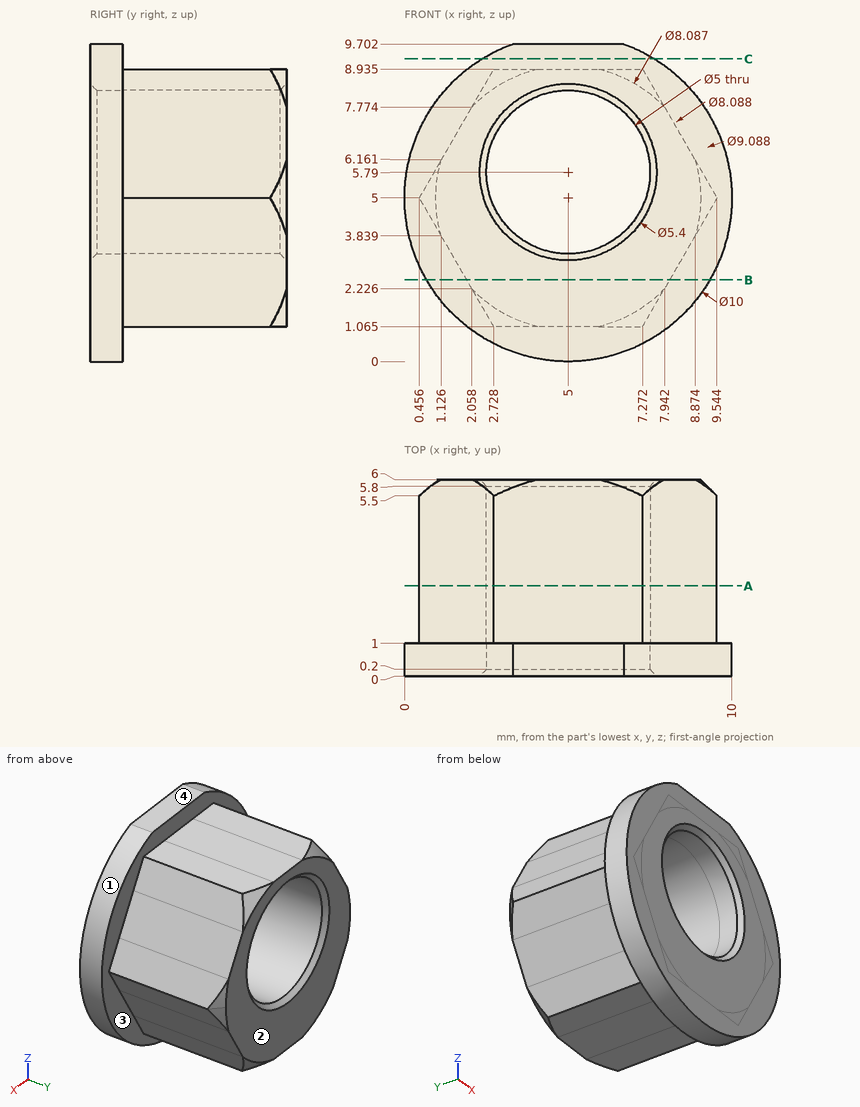
Can you work these out from the drawing? Everything is in mm from the part's minimum corner. A direction names the side the tool comes from. Coordinates: 2 decimals unless noted, no trailing zeros. Loops run counter-clockwise (first coordinate to the right, second up) from the corner with the lowest first, then second, coordinate; pieces in that order, holes last. Notation, with made-up numbers: (7.25, 88) -> (36.25, 88) arc R15 cw to (36.25, 111) -> close; hole circle Ø6 at (4.5, -8). An arc over 180 degrees is marked (long way). Return JSON: item names as keys, results as strings.
1) If we section it at A-A, the plane y = 2.75: Write out the boundary of the cut face in (x, z) (1 decimal).
Results below:
{"outline": "(0.5, 5) -> (1.1, 3.8) -> (2.1, 2.2) -> (2.7, 1.1) -> (7.3, 1.1) -> (7.9, 2.2) -> (8.9, 3.8) -> (9.5, 5) -> (8.9, 6.2) -> (7.9, 7.8) -> (7.3, 8.9) -> (2.7, 8.9) -> (2.1, 7.8) -> (1.1, 6.2) -> close; hole circle Ø5 at (5, 5.8)"}
2) For the marked faces 3 and 4, which set-ups out of +Z, -Z, +X, -X, +Y, -Y let a thin tool reach every point of the face, with its end or its side?
Results below:
{"face 3": "+Y", "face 4": "+Z, +X, -X, +Y, -Y"}
3) Thinking about a two-plate mould opening in Y: for the marked faces 1 and 2, which applies, +Y half, -Y half, draft (parallel to the pull), parting line (faces both ways), or undercut?
Results below:
{"face 1": "draft", "face 2": "+Y half"}
4) If we section it at B-B, the plane z = 2.5: Write out the boundary of the cut face in (x, y).
Results below:
{"outline": "(0.67, 0) -> (9.33, 0) -> (9.33, 1) -> (8.1, 1) -> (8.1, 6) -> (1.9, 6) -> (1.9, 1) -> (0.67, 1) -> close"}
5) I need wall thicknesses on line 1 (X direction, y = 0.5, z = 5.75); line 2 (Z direction, x = 6, y = 1.5) (1 decimal); line 3 (X direction, y = 4.25, z = 4.5) (1 decimal). Which ranges of each line are inside material? Lowest first, please. Write a range as from..to.
Results below:
{"line 1": "0.06..2.5, 7.5..9.94", "line 2": "1.1..3.5, 8.1..8.9", "line 3": "0.7..2.9, 7.1..9.3"}
6) Will these pins go through, and if not, where does the flat tip stop? pin 1 (1 mm diameter, centred on x = 3, y = 4, fed in from +Z) (1 decimal); pin 2 (3 mm diameter, centred on x = 6.5, z = 4.5, fed in from +Y); pin 3 (1.5 mm diameter, centred on x = 3.5, y = 2.5, fed in from -Z) (1 decimal); pin 4 (3 mm diameter, centred on x = 1.5, y = 1.5, fed in from -Z) (1 decimal).
Results below:
{"pin 1": "z = 8.9", "pin 2": "y = 6", "pin 3": "z = 1.1", "pin 4": "z = 0.5"}
7) If we section it at C-C, the plane z = 9.25: Write out the boundary of the cut face in (x, y).
Results below:
{"outline": "(2.37, 0) -> (7.63, 0) -> (7.63, 1) -> (2.37, 1) -> close"}
